Autodesk Inventor part; units mm, degrees
ref_plane "YZ Plane" through (0, 0, 0) normal (1, 0, 0) x (0, 1, 0)
ref_plane "XZ Plane" through (0, 0, 0) normal (0, 1, 0) x (-1, 0, 0)
ref_plane "XY Plane" through (0, 0, 0) normal (0, 0, 1) x (1, 0, 0)
sketch "Sketch1" plane through (0, 0, 0) normal (0, 1, 0) x (-1, 0, 0)
  line L0 (20, 20) -> (20, -20)
  line L1 (20, -20) -> (-20, -20)
  line L2 (-20, -20) -> (-20, 0)
  line L3 (20, 20) -> (0, 20)
  line L4 (0, 20) -> (-20, 0)
  point P0 (0, 0)
  point P1 (0, -20)
  point P2 (20, 0)
  dimension "d0" = 40
  dimension "d1" = 40
  dimension "d2" = 20
  dimension "d3" = 20
extrude "Extrusion1" add sketch "Sketch1" along normal blind 3
sketch "Sketch2" plane through (0, 3, 0) normal (0, 1, 0) x (1, 0, 0)
  line L0 (-20, 20) -> (-20, -20)
  line L1 (20, 0) -> (20, 20)
  line L2 (20, 20) -> (-20, 20)
  point P0 (0, 0)
  point P1 (-10, 10)
  point P2 (10, 10)
  dimension "d6" = 10
  dimension "d7" = 10
  dimension "d8" = 10
hole "Hole1" at (-10, 3, -10) at (10, 3, -10) direction (0, -1, 0) diameter 4.5 end through all
sketch "Sketch3" plane through (0, 3, 0) normal (0, 1, 0) x (1, 0, 0)
  line L0 (-20, -20) -> (0, -20)
  line L1 (-20, 20) -> (-20, -20)
  point P0 (0, 0)
  point P1 (-10, -10)
  dimension "d16" = 10
  dimension "d17" = 10
hole "Hole2" at (-10, 3, 10) direction (0, -1, 0) diameter 5.5 end through all
equation "\"d1\" = d0"
properties part number "X-Axis End - Corner"
Source: CAD feature listing. Evaluate the final solid. Frame: model axes, mm. Round coordinates to 2 decimals unless told otherwise and drop trailing zeros. Write each loop counter-clockwise with the first axis right and the second up, starting at its lowest first coordinate (ties: lowest second). Pieces come first, ordered by that corner, then holes. Notation, with made-up numbers: M 21,7 L 44,7 A22 ccw 44,26 Z; hole C 20,69 d4. An arc over 180 degrees is marked long. Answer as a JSON object with one key per item and string values. Group by question number.
(1) Section query A-A on x = -10. Output: boundary loops of the cut face in (y, z), then the cut area to 3 significant figures.
(2) Ray query, line 1 (X direction, y = 2, z = -10); line 2 (Z direction, x = -10, y = 1.4); line 3 (Z direction, x = 10, y = 1.75). Return the intervals inside material, ascending. Write a range as [from, to].
(3) Section query B-B on z = 10. Output: boundary loops of the cut face in (x, y), then the cut area to 3 significant figures.
(4) Mould query, pull axis Z, two halves, no side actions, for faces 1 (the cylindrical face through (-12.32, 1.48, 11.48)), 2 (the flat face through (-10, 1, 20)), 3 (the cylindrical face through (-11.52, 1.48, -11.66)), 4 (the flat face through (0, 0, 0)). Classes: +Z half, -Z half, draft (parallel to the pull), parting line (faces both ways), or undercut.
(5) First-contact query: pin 1 (1 mm diameter, centred on y = 1, z = 14, fed in from +X); pin 2 (9 mm diameter, centred on x = -10, z = 10, fed in from -Y). Flat tips, straight axial feed; report the tip coordinate or a pass-through.
(6) Section query C-C on x = 10. Output: boundary loops of the cut face in (y, z), then the cut area to 3 significant figures.
(7) Section query D-D on y = 1.9. Output: boundary loops of the cut face in (x, z), then the cut area to 3 significant figures.
Computed values:
{
 "1": {"outline": "M 0,-20 L 3,-20 L 3,-12.25 L 0,-12.25 Z; M 0,-7.75 L 3,-7.75 L 3,7.25 L 0,7.25 Z; M 0,12.75 L 3,12.75 L 3,20 L 0,20 Z", "area": "90.0 mm^2"},
 "2": {"line 1": "[-20, -12.25], [-7.75, 7.75], [12.25, 20]", "line 2": "[-20, -12.25], [-7.75, 7.25], [12.75, 20]", "line 3": "[-20, -12.25], [-7.75, 10]"},
 "3": {"outline": "M -20,0 L -12.75,0 L -12.75,3 L -20,3 Z; M -7.25,0 L 10,0 L 10,3 L -7.25,3 Z", "area": "73.5 mm^2"},
 "4": {"face 1": "undercut", "face 2": "+Z half", "face 3": "undercut", "face 4": "draft"},
 "5": {"pin 1": "x = 6.5", "pin 2": "y = 0"},
 "6": {"outline": "M 0,-20 L 3,-20 L 3,-12.25 L 0,-12.25 Z; M 0,-7.75 L 3,-7.75 L 3,10 L 0,10 Z", "area": "76.5 mm^2"},
 "7": {"outline": "M -20,-20 L 20,-20 L 20,0 L 0,20 L -20,20 Z; hole C -10,10 d5.5; hole C -10,-10 d4.5; hole C 10,-10 d4.5", "area": "1,340 mm^2"}
}
